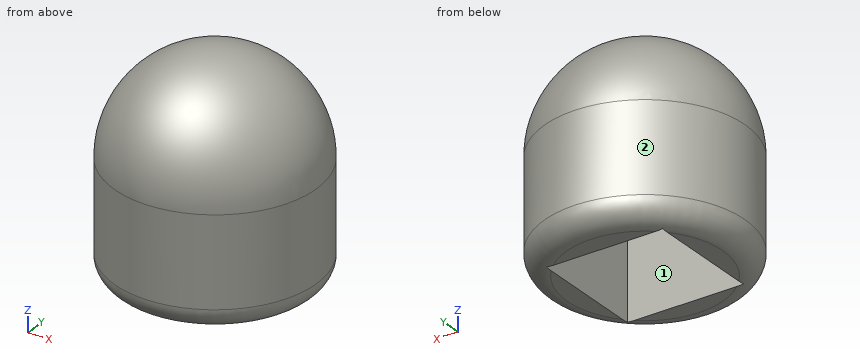
from build123d import *

# Parameters (mm, degrees)
SKETCH_3_R          = 9
EXTRUDE_1_DEPTH     = 10
SKETCH_2_W          = 10.5
SKETCH_2_H          = 10.5
CUT_EXTRUDE_1_DEPTH = 10
FILLET_1_R          = 2


with BuildPart() as part:
    # 草图1 → 旋转1 (revolve)
    with BuildSketch(Plane.XY):
        with BuildLine():
            Line((0, 9), (0, -9))
            ThreePointArc((0, -9), (9, 0), (0, 9))
        make_face()
    revolve(axis=Axis((0, 9, 0), (0, -1, 0)))

    # 草图3 → 凸台-拉伸1 (add)
    with BuildSketch(Plane.XY):
        Circle(SKETCH_3_R)
    extrude(amount=-EXTRUDE_1_DEPTH)

    # 草图2 → 切除-拉伸1 (cut)
    with BuildSketch(Plane.XY):
        Rectangle(SKETCH_2_W, SKETCH_2_H)
    extrude(amount=-CUT_EXTRUDE_1_DEPTH, mode=Mode.SUBTRACT)

    # 圆角1
    # the kernel refuses this fillet: 2 mm, written as the material it takes off along each edge
    with BuildSketch(Plane(origin=(0, 0, -10), x_dir=(1, 0, 0), z_dir=(0, -1, 0))) as fillet_1_piece_1:
        with BuildLine():
            CenterArc((9 - FILLET_1_R, FILLET_1_R), FILLET_1_R, 270, 90)
            Line((9 - FILLET_1_R, 0), (9, 0))
            Line((9, 0), (9, FILLET_1_R))
        make_face()
    revolve(axis=Axis((0, 0, -10), (0, 0, 1)), mode=Mode.SUBTRACT)


solid = part.part
Here's how the part is built. I have some questions about the finished solid (model axes, mm). Face numbers are marked on the shaded views. Coordinates: 2 decimals unless noted, no trailing zeros. Loops run counter-clockwise (first coordinate to the right, second up) from the corner with the lowest first, then second, coordinate; pieces in that order, holes last. Notation, with made-up numbers: (56.25, -8.5) -> (84.25, -8.5) arc R18 cw to (84.25, -4.5) -> close; hole circle Ø3 at (41.5, 73.5). An arc over 180 degrees is marked (long way). Use one line per item in the form item = value. Start each with the question number.
(1) If we section it at A-A (y = 0): Please give me the cut outline in (x, z), then the cut area to 3 significant figures.
(2) We'd pull the mould along X, two halves only. Please class the marked faces 1 and 2: pulls with the +X half, pulls with the -X half, needs draft (parallel to the pull), parting line crosses it, or undercut.
(3) If we section it at D-D (z = 5.25): Please give me the cut outline in (x, y), then the cut area to 3 significant figures.
(4) Please list where these lines run through material, in increasing order: line 1 along Y through (x, z) = (-1.75, -7.75); line 2 along Y through (x, z) = (-2.75, -5.75); line 3 along Z through (x, y) = (2.25, -3).
(5) If we section it at C-C (z = -2.75): Please give me the cut outline in (x, y), then the cut area to 3 significant figures.
(6) Will these pins go through, and if not, where does the flat tip stop? pin 1 (3 mm diameter, centred on x = 1, y = -1, fed in from -Z); pin 2 (3 mm diameter, centred on x = 2, z = -4.5, fed in from +Y); pin 3 (4 mm diameter, centred on y = -7, z = -3, fed in from +X).
Verdict:
q1.outline = (-9, -8) arc R2 ccw to (-7, -10) -> (-5.25, -10) -> (-5.25, 0) -> (5.25, 0) -> (5.25, -10) -> (7, -10) arc R2 ccw to (9, -8) -> (9, 0) arc R9 ccw to (-9, 0) -> close
q1.area = 201 mm²
q2.face_1 = undercut
q2.face_2 = parting line crosses it
q3.outline = circle Ø14.62 at (0, 0)
q3.area = 168 mm²
q4.line_1 = -8.83 to -5.25, 5.25 to 8.83
q4.line_2 = -8.57 to -5.25, 5.25 to 8.57
q4.line_3 = 0 to 8.18
q5.outline = circle Ø18 at (0, 0); hole (-5.25, -5.25) -> (5.25, -5.25) -> (5.25, 5.25) -> (-5.25, 5.25) -> close
q5.area = 144 mm²
q6.pin_1 = 0
q6.pin_2 = 8.99
q6.pin_3 = 7.48
